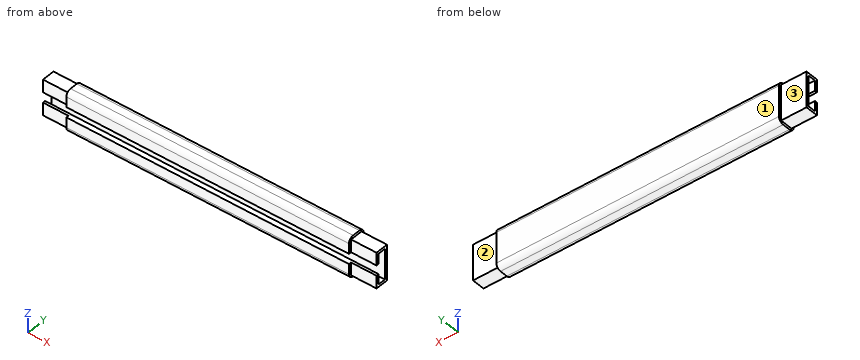
from build123d import *

# Parameters (mm, degrees)
F0_W     = 121
F0_H     = 16
F1_DEPTH = 7
F3_DEPTH = 121.001
F5_DEPTH = 10
F7_DEPTH = 10
F8_R     = 2


with BuildPart() as f1:
    # F0 (on Front) → F1 (new body)
    with BuildSketch(Plane.XZ):
        with Locations((40.8839493543, 17.2579787597)):
            Rectangle(F0_W, F0_H)
    extrude(amount=F1_DEPTH)

    # F2 (on face) → F3 (cut, through all)
    with BuildSketch(Plane.YZ.offset(101.3839493543)):
        Polygon((-7, 19.2579787597), (-7, 15.2579787597), (-5, 15.2579787597), (-5, 11.2579787597), (-2, 11.2579787597), (-2, 23.2579787597), (-5, 23.2579787597), (-5, 19.2579787597), align=None)
    extrude(amount=-F3_DEPTH, mode=Mode.SUBTRACT)

    # F4 (on face) → F5 (join)
    with BuildSketch(Plane.YZ.offset(101.3839493543)):
        Polygon((-6, 15.2579787597), (-6, 10.2579787597), (-1, 10.2579787597), (-1, 24.2579787597), (-6, 24.2579787597), (-6, 19.2579787597), (-5, 19.2579787597), (-5, 23.2579787597), (-2, 23.2579787597), (-2, 11.2579787597), (-5, 11.2579787597), (-5, 15.2579787597), align=None)
    extrude(amount=F5_DEPTH)

    # F6 (on face) → F7 (cut)
    with BuildSketch(Plane(origin=(-19.6160506457, 0, 0), x_dir=(0, -1, 0), z_dir=(-1, 0, 0))):
        Polygon((1, 24.2579787597), (6, 24.2579787597), (6, 19.2579787597), (7, 19.2579787597), (7, 25.2579787597), (0, 25.2579787597), (0, 9.2579787597), (7, 9.2579787597), (7, 15.2579787597), (6, 15.2579787597), (6, 10.2579787597), (1, 10.2579787597), align=None)
    extrude(amount=-F7_DEPTH, mode=Mode.SUBTRACT)

    # F8
    f8_edges = [f1.edges().sort_by_distance(p)[0] for p in [
        (45.883949, -7, 25.257979),
        (45.883949, -7, 9.257979),
        (45.883949, 0, 25.257979),
        (45.883949, 0, 9.257979),
    ]]
    fillet(f8_edges, radius=F8_R)


solid = f1.part
Geometry check sheet. Reference: the model listing, model coordinates, mm. Face numbers are marked on the shaded views. A direction names the side the tool comes from. Round coordinates to 2 decimals unless told otherwise and drop trailing zeros. Loops run counter-clockwise (first coordinate to the right, second up) from the corner with the lowest first, then second, coordinate; pieces in that order, holes last. Notation, with made-up numbers: (43, 4) -> (61, 4) arc R23 cw to (61, 31) -> close; hole circle Ø8 at (76, 61.25). An arc over 180 degrees is marked (long way). Answer as a JSON object with one key per item and string values. Group by question number.
Item 1: Thickness scan on line 1 along Y through (x, z) = (31, 15); line 2 along Z through (x, y) = (-7.5, -5.25); line 3 along Y through (x, z) = (106, 12). Record the ranges inside material, lowest first.
Item 2: Cross-section at D-D, the plane z = 18. Record the cut outline in (x, y).
Item 3: Cross-section at A-A, the plane y = -3.75. Record the cut outline in (x, z).
Item 4: Cross-section at B-B, the plane z = 13.25. Record the cut outline in (x, y).
Item 5: Set-up check for the marked faces 1, 2 and 3: record each of +Z, -Z, +X, -X, +Y, -Y from which the full face is reachable in a straight line by a thin tool's end or side.
Item 6: Cross-section at C-C, the plane x = 67. Record the cut outline in (y, z), plus the area to 3 significant figures.
Item 7: Depth check by flat-ended pin: pin 1 Ø1 at (x, y) = (20.5, -6) entering from -Z; pin 2 Ø1.5 at (x, y) = (-13.5, -3) entering from +Z; pin 3 Ø1.5 at (x, z) = (104, 22) entering from -Y. Enter the tip coordinate at first touch or a pass-through.
Determined:
{
 "1": {"line 1": "y = -7 to -5, -2 to 0", "line 2": "z = 9.27 to 15.26, 19.26 to 25.24", "line 3": "y = -6 to -5, -2 to -1"},
 "2": {"outline": "(-19.62, -2) -> (111.38, -2) -> (111.38, -1) -> (101.38, -1) -> (101.38, 0) -> (-9.62, 0) -> (-9.62, -1) -> (-19.62, -1) -> close"},
 "3": {"outline": "(-19.62, 10.26) -> (-9.62, 10.26) -> (-9.62, 9.26) -> (101.38, 9.26) -> (101.38, 10.26) -> (111.38, 10.26) -> (111.38, 11.26) -> (-19.62, 11.26) -> close; (-19.62, 23.26) -> (111.38, 23.26) -> (111.38, 24.26) -> (101.38, 24.26) -> (101.38, 25.26) -> (-9.62, 25.26) -> (-9.62, 24.26) -> (-19.62, 24.26) -> close"},
 "4": {"outline": "(-19.62, -6) -> (-9.62, -6) -> (-9.62, -7) -> (101.38, -7) -> (101.38, -6) -> (111.38, -6) -> (111.38, -5) -> (-19.62, -5) -> close; (-19.62, -2) -> (111.38, -2) -> (111.38, -1) -> (101.38, -1) -> (101.38, 0) -> (-9.62, 0) -> (-9.62, -1) -> (-19.62, -1) -> close"},
 "5": {"face 1": "+Z, -Z, +X, -X, +Y", "face 2": "+Z, -Z, +X, +Y", "face 3": "+Z, -Z, -X, +Y"},
 "6": {"outline": "(-7, 11.26) arc R2 ccw to (-5, 9.26) -> (-2, 9.26) arc R2 ccw to (0, 11.26) -> (0, 23.26) arc R2 ccw to (-2, 25.26) -> (-5, 25.26) arc R2 ccw to (-7, 23.26) -> (-7, 19.26) -> (-5, 19.26) -> (-5, 23.26) -> (-2, 23.26) -> (-2, 11.26) -> (-5, 11.26) -> (-5, 15.26) -> (-7, 15.26) -> close", "area": "64.6 mm²"},
 "7": {"pin 1": "stops at z = 9.32", "pin 2": "stops at z = 24.26", "pin 3": "stops at y = -6"}
}
